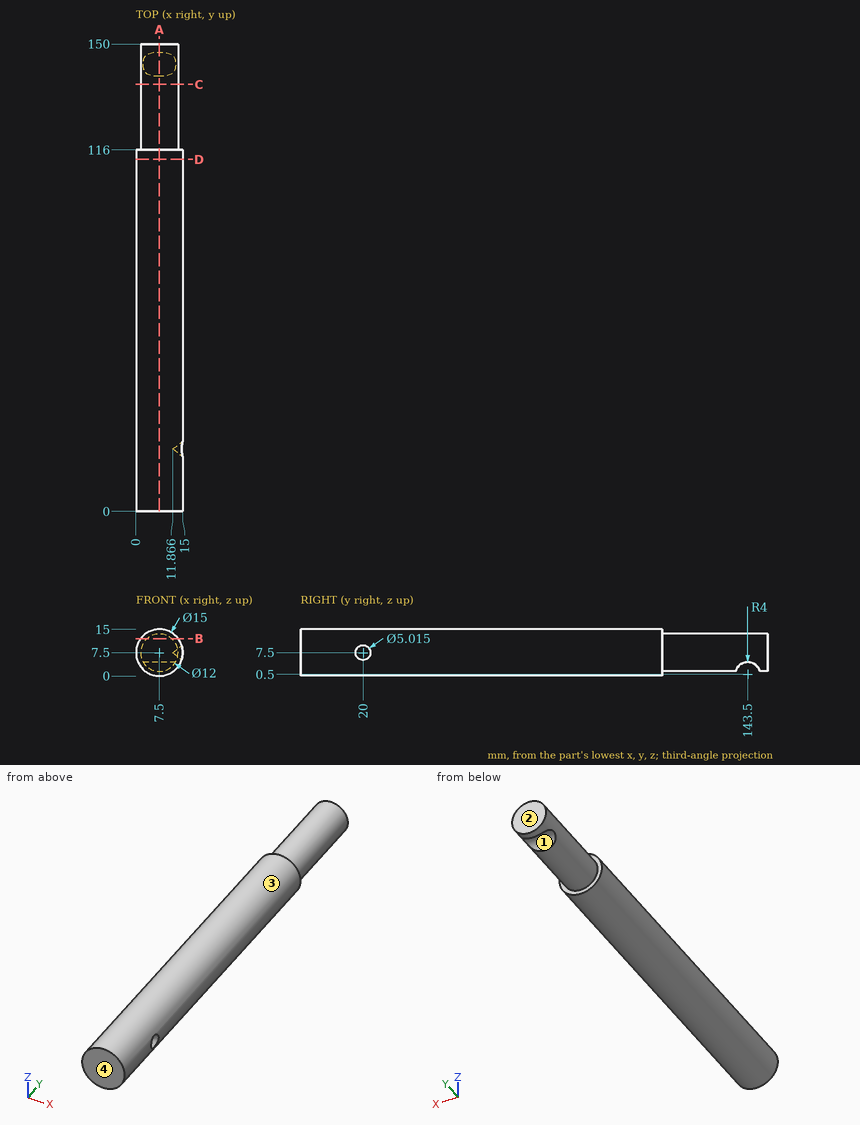
The figure shows three views and two pictorial views of one solid part (mm, origin at its lowest corner). Answer the questions. Round coordinates to 2 decimals unless told otherwise and drop trailing zeros. Order: outer loops, then holes, each group sorted by start corner. A loop starts at its lowest first (then second) coordinate and runs counter-clockwise, first axis right, second up. Notation, with made-up numbers: M -10,-34 L -1,-34 A13 cw -1,-26 Z; hole C -31.5,54 d11. An arc over 180 degrees is marked long. Answer in a Markdown table with one row per item. Add a question column.
1) Consider line 1 along Z through (x, y) = (7, 44); line 2 along Y through (x, z) = (11.5, 12.5); line 3 along Y through (x, z) = (11, 3.5) (1 decimal). Determine where each line is inside the solid, lowest interval first. Write a range as from..to.
2) Flat-ended cylindrical pins translate along their axes: pin 1 Ø1.5 at (y, z) = (82, 2) entering from +X (1 decimal); pin 2 Ø1.5 at (y, z) = (126.5, 5) entering from +X; pin 3 Ø4 at (y, z) = (133, 9.5) entering from +X. Find the tip coordinate at first contact, or state that the pin passes through.
3) The part is cut by section A-A on x = 7.5. Determine the outline of the cut face in (y, z).
4) The part is cut by section B-B on z = 12. Determine the outline of the cut face in (x, y).
5) The part is cut by section C-C on y = 137. Determine the outline of the cut face in (x, z), plus the area to 3 significant figures.
6) The part is cut by section D-D on y = 113. Determine the outline of the cut face in (x, z), plus the area to 3 significant figures.
7) Determine the mould class of the marked faces 1, 2, 3 and 4 for opening direction Y: pulls with the +Y half, pulls with the -Y half, needs draft (parallel to the pull), parting line crosses it, or undercut.
Findings below:
| question | item | result |
|---|---|---|
| 1 | line 1 | z = 0.02..14.98 |
| 1 | line 2 | y = 0..116 |
| 1 | line 3 | y = 0..140.9, 146.1..150 |
| 2 | pin 1 | stops at x = 13.3 |
| 2 | pin 2 | stops at x = 13.24 |
| 2 | pin 3 | stops at x = 13.5 |
| 3 | outline | M 0,0 L 116,0 L 116,1.5 L 139.63,1.5 A4 cw 147.37,1.5 L 150,1.5 L 150,13.5 L 116,13.5 L 116,15 L 0,15 Z |
| 4 | outline | M 1.5,0 L 13.5,0 L 13.5,116 L 11.47,116 L 11.47,150 L 3.53,150 L 3.53,116 L 1.5,116 Z |
| 5 | outline | C 7.5,7.5 d12 |
| 5 | area | 113 mm² |
| 6 | outline | C 7.5,7.5 d15 |
| 6 | area | 177 mm² |
| 7 | face 1 | undercut |
| 7 | face 2 | pulls with the +Y half |
| 7 | face 3 | needs draft |
| 7 | face 4 | pulls with the -Y half |
